Verification items for the finished model (mm, model axes). A direction names the side the tool comes from. Coordinates: 2 decimals unless noted, no trailing zeros. Loops run counter-clockwise (first coordinate to the right, second up) from the corner with the lowest first, then second, coordinate; pieces in that order, holes last.
Q1. Mould release check, pull along X, two halves, no side actions. Record for faces 1 (the face through (-47.08, 17.55, 91.95)), 2 (the face through (-37, 13, 0)), 3 (the face through (-37.751, 33.842, 87.655)): +X half, -X half, draft (parallel to the pull), parting line (faces both ways), or undercut.
Q2. Access from +Z, -Z, +X, -X, +Y, -Y to the whole of each face (thin tool, end or side, straight path). Record for faces 4 (the face through (-26.874, 18.54, 91.948)), 5 (the face through (-24.84, -0.12, 87.66)).
Q3. Sectioned sample at D-D (y = 28.5). Enter the section's corners in (x, z).
Q4. Sectioned sample at B-B (x = -26). Enter the section's corners in (y, z), then the cut area to 3 significant figures.
Q5. Sectioned sample at A-A (z = 14). Enter the section's corners in (x, y).
Q6. Go/stop test with flat-tipped pins: P1, Ø3, axis at x = -30, z = 30.5, coming from the +Y side; P2, Ø4, axis at y = 15, z = 93, coming from the +X side; P3, Ø4, axis at y = 13, z = 26.5, coming from the -X side. Record where each tip stops, or that it passes through.
Q7. Material ranges on probe 1 along Y at (x, z) = (-43, 64.5); probe 2 along X at (y, z) = (2, 146); probe 3 along Z at (x, y) = (-34, 25), recorded low to high.
Q8. Sectioned sample at C-C (y = 19). Enter the section's corners in (x, z), then the cut area to 3 significant figures.
```python
from build123d import *

# Parameters (mm, degrees)
F1_DEPTH = 177.8
F2_T     = -8.4666666667


# Not quite as in the source:
# - a length typed as a fraction of an inch, garbled in the dataset ("3 / 203.2 mm" for 3/8 in), is restored


with BuildPart() as f1:
    # F0 (on Top) → F1 (new body)
    with BuildSketch(Plane.XY):
        Polygon((-35.4204343678, -8.8066042373), (-13.96876778, 8.8066042373), (-24.0909949393, 34.6511322751), (-51.7985419534, 33.0107205511), (-58.8005205937, 6.1523623123), align=None)
    extrude(amount=F1_DEPTH)

    # F2
    f2_openings = [f1.faces().sort_by_distance(p)[0] for p in [
        (-36.815852, 14.762843, 177.8),
    ]]
    offset(amount=F2_T, openings=f2_openings)


solid = f1.part
```
Geometry check:
1. face 1: undercut
1. face 2: draft
1. face 3: -X half
2. face 4: +Z
2. face 5: +Z, -Z, +X, -Y
3. outline: (-52.97, 0) - (-21.68, 0) - (-21.68, 177.8) - (-52.97, 177.8) - close
4. outline: (-1.07, 0) - (34.54, 0) - (34.54, 177.8) - (16.31, 177.8) - (16.31, 8.47) - (9.88, 8.47) - (9.88, 177.8) - (-1.07, 177.8) - close
4. area: 5,240 mm2
5. outline: (-58.8, 6.15) - (-35.42, -8.81) - (-13.97, 8.81) - (-24.09, 34.65) - (-51.8, 33.01) - close; hole (-49.06, 9.97) - (-36.04, 1.64) - (-24.1, 11.45) - (-29.73, 25.84) - (-45.16, 24.92) - close
6. P1: stops at y = 34.39
6. P2: stops at x = -15.61
6. P3: stops at x = -57.54
7. probe 1: y = -3.96 to 6.09, 25.05 to 33.53
7. probe 2: x = -52.31 to -36.6, -35.6 to -22.26
7. probe 3: z = 0 to 8.47
8. outline: (-55.45, 0) - (-17.96, 0) - (-17.96, 177.8) - (-27.05, 177.8) - (-27.05, 8.47) - (-46.7, 8.47) - (-46.7, 177.8) - (-55.45, 177.8) - close
8. area: 3,340 mm2
